Autodesk Inventor part; units mm, degrees
ref_plane "YZ Plane" through (0, 0, 0) normal (1, 0, 0) x (0, 1, 0)
ref_plane "XZ Plane" through (0, 0, 0) normal (0, 1, 0) x (-1, 0, 0)
ref_plane "XY Plane" through (0, 0, 0) normal (0, 0, 1) x (1, 0, 0)
sketch "Sketch1" plane through (0, 0, 0) normal (1, 0, 0) x (0, 1, 0)
  line L0 (0, 0) -> (-25, 0)
  line L1 (-25, 0) -> (-25, -40)
  line L2 (-25, -40) -> (0, -40)
  line L3 (0, -40) -> (0, 0)
  dimension "d0" = 25
  dimension "d1" = 40
extrude "Extrusion1" add sketch "Sketch1" along normal blind 20
sketch "Sketch2" plane through (20, 0, 0) normal (1, 0, 0) x (0, 0, -1)
  line L0 (0, 0) -> (20, 0)
  line L1 (40, 0) -> (0, 0)
  line L2 (20, 0) -> (20, -10)
  circle A0 centre (20, -10) radius 2.5
  dimension "d4" = 20
  dimension "d5" = 10
  dimension "d6" = 5
extrude "Extrusion2" cut sketch "Sketch2" against normal blind 20
sketch "Sketch3" plane through (0, 0, 0) normal (0, 1, 0) x (1, 0, 0)
  line L0 (0, 0) -> (20, 0)
  line L1 (0, 0) -> (10, 0)
  line L2 (10, 0) -> (10, 6)
  line L3 (0, 40) -> (10, 40)
  line L4 (0, 40) -> (20, 40)
  line L5 (10, 40) -> (10, 34)
  circle A0 centre (10, 6) radius 2.5
  circle A1 centre (10, 34) radius 2.5
  dimension "d9" = 10
  dimension "d10" = 6
  dimension "d11" = 6
  dimension "d12" = 5
  dimension "d13" = 5
extrude "Extrusion3" cut sketch "Sketch3" against normal through all
sketch "Sketch4" plane through (0, 0, 0) normal (-1, 0, 0) x (0, 0, 1)
  circle A0 centre (-20, -10) radius 2.5
  circle A1 centre (-20, -10) radius 8
  point P0 (0, 0)
  dimension "d16" = 16
extrude "Extrusion4" cut sketch "Sketch4" against normal blind 9.5
sketch "Sketch5" plane through (9.5, -10, -20) normal (-1, 0, 0) x (0, 0, 1)
  circle A0 centre (0, 0) radius 3
  point P0 (20, 10)
  dimension "d19" = 6
extrude "Extrusion5" cut sketch "Sketch5" against normal through all
sketch "Sketch6" plane through (0, 0, 0) normal (-1, 0, 0) x (0, 0, 1)
  line L0 (-57.9528, 15.7727) -> (32.6208, 15.7727)
  line L1 (32.6208, 15.7727) -> (32.6208, -49.7079)
  line L2 (32.6208, -49.7079) -> (-57.9528, -49.7079)
  line L3 (-57.9528, -49.7079) -> (-57.9528, 15.7727)
  point P0 (0, 0)
extrude "Extrusion6" cut sketch "Sketch6" against normal blind 3.5
properties part number "linac_mover_upper_ax_holder"
Build history of the part. All positions in model axes, mm. A direction names the side the tool comes from. Coordinates: 2 decimals unless noted, no trailing zeros. Write each loop counter-clockwise with the first axis right and the second up, starting at its lowest first coordinate (ties: lowest second). Pieces come first, ordered by that corner, then holes. Notation, with made-up numbers: (38, 74.5) -> (88, 74.5) arc R24 ccw to (88, 98.5) -> close; hole circle Ø6 at (79.5, 57). An arc over 180 degrees is marked (long way). Use CSV: the item, a comma, the result in double quotes. Start each with the question number.
Q1. 3-axis set-ups, long thin cutter, end or side, ignore diameter. For faces 4 (the cylindrical face through (15, -10, -23)), 5 (the flat face through (9.5, -13.4, -20.1)): which of +Z, -Z, +X, -X, +Y, -Y reach the whole face in a straight line?
Q2. Drill centre lines: probe 1 along Y at (x, z) = (15, -20); probe 2 along Z at (x, y) = (7.75, -9.5); probe 3 along Z at (x, y) = (10, -13.75). Where is each one in solid material? Low to high.
Q3. Flat gauge pins, fed straight in: pin 1 Ø8 at (y, z) = (-12.5, -22) entering from -X; pin 2 Ø7 at (y, z) = (-10, -20) entering from +X. Where does each tip first touch, or does it go through?
Q4. Cut at A-A, the plane x = 10. List the corners of the cut face in (y, z), then the cut area to 3 significant figures.
Q5. Pull direction Z, two halves, no side cores. Call faces 1 (the cylindrical face through (6.458, -14.868, -26.349)), 2 (the flat face through (3.5, -18, -16)), 3 (the flat face through (12, -13, -40)): released by +Z, released by -Z, zero draft, split by the parting line, or undercut.
Q6. Cut at D-D, the plane x = 8. List the corners of the cut face in (y, z).
Q7. Cut at B-B, the plane y = -10. List the corners of the cut face in (x, z).
Q8. Cut at C-C, the plane z = -6. List the corners of the cut face in (x, y), then the cut area to 4 significant figures.
Checked values:
1,face 4,"+X, -X"
1,face 5,"-X"
2,probe 1,"y = -25 to -13, -7 to 0"
2,probe 2,"z = -40 to -35.09, -32.91 to -27.98, -12.02 to -7.09, -4.91 to 0"
2,probe 3,"z = -40 to -36.5, -31.5 to -8.5, -3.5 to 0"
3,pin 1,"stops at x = 9.5"
3,pin 2,"stops at x = 20"
4,outline,"(-25, -40) -> (0, -40) -> (0, -36.5) -> (-25, -36.5) -> close; (-25, -31.5) -> (0, -31.5) -> (0, -8.5) -> (-25, -8.5) -> close; (-25, -3.5) -> (0, -3.5) -> (0, 0) -> (-25, 0) -> close; hole circle Ø6 at (-10, -20)"
4,area,"722 mm²"
5,face 1,"undercut"
5,face 2,"zero draft"
5,face 3,"released by -Z"
6,outline,"(-25, -40) -> (0, -40) -> (0, -35.5) -> (-25, -35.5) -> close; (-25, -32.5) -> (0, -32.5) -> (0, -7.5) -> (-25, -7.5) -> close; (-25, -4.5) -> (0, -4.5) -> (0, 0) -> (-25, 0) -> close; hole circle Ø16 at (-10, -20)"
7,outline,"(3.5, -40) -> (20, -40) -> (20, -23) -> (9.5, -23) -> (9.5, -28) -> (3.5, -28) -> close; (3.5, -12) -> (9.5, -12) -> (9.5, -17) -> (20, -17) -> (20, 0) -> (3.5, 0) -> close; hole circle Ø5 at (10, -34); hole circle Ø5 at (10, -6)"
8,outline,"(3.5, -25) -> (7.5, -25) -> (7.5, 0) -> (3.5, 0) -> close; (12.5, -25) -> (20, -25) -> (20, 0) -> (12.5, 0) -> close"
8,area,"287.5 mm²"
